Input: part model. Units: mm. Frame: model coordinates. Coordinates: 2 decimals unless noted, no trailing zeros. Write each loop counter-clockwise with the first axis right and the second up, starting at its lowest first coordinate (ties: lowest second). Pieces come first, ordered by that corner, then holes.
1) Section query A-A (y = 0). Output: boundary loops of the cut face in (x, z), then the cut area to 3 significant figures.
2) Line query: L1, parallel to Y at x = 125, z = -0.75; L2, parallel to X at y = 0.25, z = -1.25; L3, parallel to X at y = -3.5, z = 1.75. Output: solid intervals per line, ascending.
3) Section query C-C (z = -0.25). Output: boundary loops of the cut face in (x, y), then the cut area to 3 significant figures.
4) Pin query (flat end, axial travel): pin 1 Ø1 at (y, z) = (-4, -2) entering from -X. Return the tip coordinate at first contact, or that it passes through.
5) Section query B-B (x = 0). Output: boundary loops of the cut face in (y, z).
from build123d import *

# Parameters (mm, degrees)
SKETCH1_R           = 5
BOSS_EXTRUDE1_DEPTH = 5
SKETCH2_R           = 5
CUT_EXTRUDE2_DEPTH  = 5


with BuildPart() as part:
    # Sketch1 → Boss-Extrude1 (new, symmetric)
    with BuildSketch(Plane.XY):
        with BuildLine():
            Line((-125, 10), (125, 10))
            ThreePointArc((125, 10), (135, 0), (125, -10))
            Line((125, -10), (-125, -10))
            ThreePointArc((-125, -10), (-135, 0), (-125, 10))
        make_face()
        with Locations((-125, 0)):
            Circle(SKETCH1_R, mode=Mode.SUBTRACT)
        with Locations((125, 0)):
            Circle(SKETCH1_R, mode=Mode.SUBTRACT)
    extrude(amount=BOSS_EXTRUDE1_DEPTH, both=True)

    # Sketch2 → Cut-Extrude2 (cut, symmetric)
    with BuildSketch(Plane.XY):
        Circle(SKETCH2_R)
    extrude(amount=CUT_EXTRUDE2_DEPTH, both=True, mode=Mode.SUBTRACT)


solid = part.part
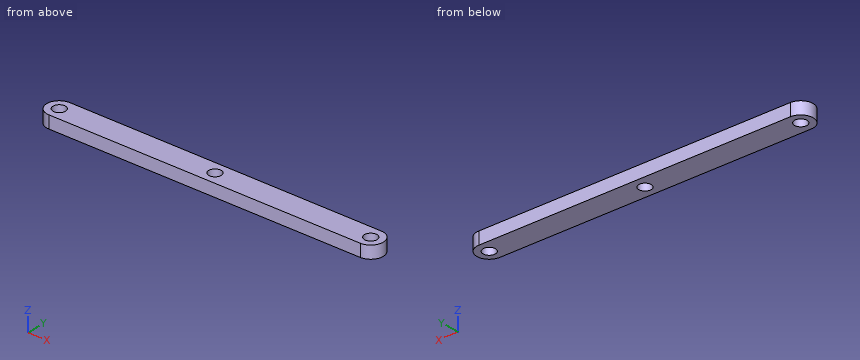
Answer:
1. outline: (-135, -5) - (-130, -5) - (-130, 5) - (-135, 5) - close; (-120, -5) - (-5, -5) - (-5, 5) - (-120, 5) - close; (5, -5) - (120, -5) - (120, 5) - (5, 5) - close; (130, -5) - (135, -5) - (135, 5) - (130, 5) - close
1. area: 2,400 mm2
2. L1: y = -10 to -5, 5 to 10
2. L2: x = -135 to -129.99, -120.01 to -4.99, 4.99 to 120.01, 129.99 to 135
2. L3: x = -134.37 to -128.57, -121.43 to -3.57, 3.57 to 121.43, 128.57 to 134.37
3. outline: (-125, -10) - (125, -10) arc R10 ccw to (125, 10) - (-125, 10) arc R10 ccw to start; hole circle Ø10 at (-125, 0); hole circle Ø10 at (0, 0); hole circle Ø10 at (125, 0)
3. area: 5,080 mm2
4. pin 1: stops at x = -134.37
5. outline: (-10, -5) - (-5, -5) - (-5, 5) - (-10, 5) - close; (5, -5) - (10, -5) - (10, 5) - (5, 5) - close
